from build123d import *

# Parameters (mm, degrees)
SKETCH1_R           = 15.5
SKETCH1_R_2         = 1.25
BOSS_EXTRUDE2_DEPTH = 12
FILLET1_R           = 2


with BuildPart() as part:
    # Sketch1 → Boss-Extrude2 (new body)
    with BuildSketch(Plane(origin=(0, 0, 0), x_dir=(1, 0, 0), z_dir=(0, 1, 0))):
        Polygon((-15, 21.000989792), (-21, 15.000989792), (-21, -15.000989792), (-15, -21.000989792), (15, -21.000989792), (21, -15.000989792), (21, 15.000989792), (15, 21.000989792), align=None)
        with Locations(Location((0, 0, 0), (0, 0, 270))):
            Circle(SKETCH1_R, mode=Mode.SUBTRACT)
        with Locations(Location((-15.5, 15.5, 0), (0, 0, 270))):
            Circle(SKETCH1_R_2, mode=Mode.SUBTRACT)
        with Locations(Location((15.5, 15.5, 0), (0, 0, 270))):
            Circle(SKETCH1_R_2, mode=Mode.SUBTRACT)
        with Locations(Location((-15.5, -15.5, 0), (0, 0, 270))):
            Circle(SKETCH1_R_2, mode=Mode.SUBTRACT)
        with Locations(Location((15.5, -15.5, 0), (0, 0, 270))):
            Circle(SKETCH1_R_2, mode=Mode.SUBTRACT)
    extrude(amount=BOSS_EXTRUDE2_DEPTH)

    # Fillet1
    fillet1_edges = [part.edges().sort_by_distance(p)[0] for p in [
        (15, 6, -21.000989792),
        (21, 6, -15.000989792),
        (21, 6, 15.000989792),
        (15, 6, 21.000989792),
        (-15, 6, 21.000989792),
        (-21, 6, 15.000989792),
        (-21, 6, -15.000989792),
        (-15, 6, -21.000989792),
    ]]
    fillet(fillet1_edges, radius=FILLET1_R)


solid = part.part
The listing builds one solid part. Answer for the finished solid, in the listing's coordinates (mm). Give positions to 0.01 mm unless a question says otherwise; leave off trailing zeros. Write each loop counter-clockwise with the first axis right and the second up, starting at its lowest first coordinate (ties: lowest second). Pieces come first, ordered by that corner, then holes.
Item 1: Find the intervals of material crossed by line 1 along Z through (x, y) = (1.5, 7.25); line 2 along X through (y, z) = (1, -11); line 3 along X through (y, z) = (2, -9), in increasing order.
Item 2: Section C-C, the plane y = 4 is taken. Write down the section's boundary in (x, z).
Item 3: Determine the mould class of faces 1 (the cylindrical face through (-20.85, 6.08, 14.93)), 2 (the cylindrical face through (-20.844, 6.084, -14.948)), 3 (the cylindrical face through (16.345, 5.916, -16.421)) for opening direction Z: released by +Z, released by -Z, zero draft, split by the parting line, or undercut.
Item 4: Section A-A, the plane x = 0 is taken. Write down the section's boundary in (y, z).
Item 5: Section B-B, the plane z = 0 is taken. Write down the section's boundary in (x, y), plus the area to 3 significant figures.
Item 6: Section D-D, the plane z = 18 is taken. Write down the section's boundary in (x, y), plus the area to 3 significant figures.
Completed:
1. line 1: z = -21 to -15.43, 15.43 to 21
1. line 2: x = -21 to -10.92, 10.92 to 21
1. line 3: x = -21 to -12.62, 12.62 to 21
2. outline: (-21, -14.17) arc R2 ccw to (-20.41, -15.59) - (-15.59, -20.42) arc R2 ccw to (-14.17, -21) - (14.17, -21) arc R2 ccw to (15.59, -20.42) - (20.41, -15.59) arc R2 ccw to (21, -14.17) - (21, 14.17) arc R2 ccw to (20.41, 15.59) - (15.59, 20.42) arc R2 ccw to (14.17, 21) - (-14.17, 21) arc R2 ccw to (-15.59, 20.42) - (-20.41, 15.59) arc R2 ccw to (-21, 14.17) - close; hole circle Ø2.5 at (-15.5, -15.5); hole circle Ø2.5 at (-15.5, 15.5); hole circle Ø31 at (0, 0); hole circle Ø2.5 at (15.5, -15.5); hole circle Ø2.5 at (15.5, 15.5)
3. face 1: released by +Z
3. face 2: released by -Z
3. face 3: undercut
4. outline: (0, -21) - (12, -21) - (12, -15.5) - (0, -15.5) - close; (0, 15.5) - (12, 15.5) - (12, 21) - (0, 21) - close
5. outline: (-21, 0) - (-15.5, 0) - (-15.5, 12) - (-21, 12) - close; (15.5, 0) - (21, 0) - (21, 12) - (15.5, 12) - close
5. area: 132 mm2
6. outline: (-18, 0) - (18, 0) - (18, 12) - (-18, 12) - close
6. area: 432 mm2
